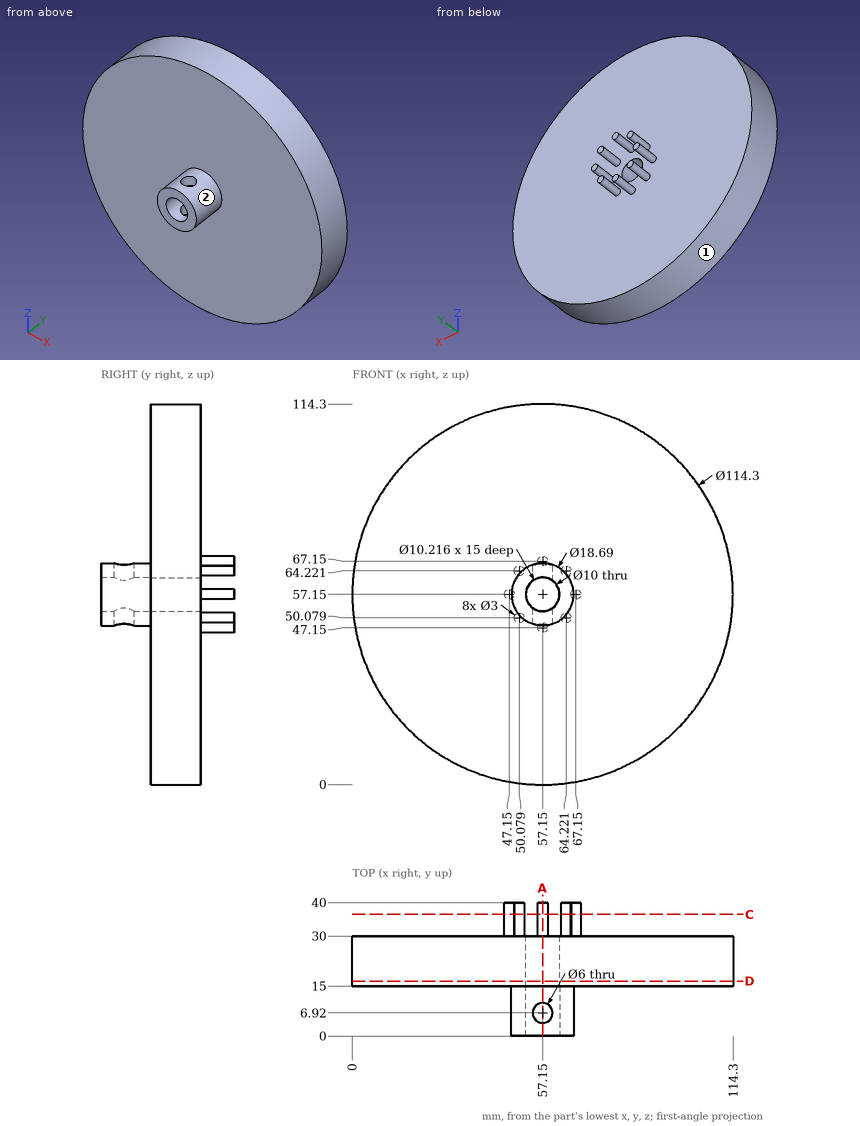
Print and shaded views of the part. All mm, measured from the part's lowest x, y and z. A direction names the side the tool comes from. Round coordinates to 2 decimals unless told otherwise and drop trailing zeros. Write each loop counter-clockwise with the first axis right and the second up, starting at its lowest first coordinate (ties: lowest second). Pieces come first, ordered by that corner, then holes.
(1) Probe line 1 along Y through (x, z) = (57.15, 49.7); line 2 along Z through (x, y) = (57, 20); line 3 along X through (y, z) = (4, 57) (1 decimal). List the from-to ranges inside material, lowest first.
(2) 3-axis set-ups, long thin cutter, end or side, ignore diameter. For the marked faces 1 and 2: which of +Z, -Z, +X, -X, +Y, -Y reach the whole face in a straight line?
(3) Drop flat-ended pins along their axis: P1, Ø6, axis at x = 57.15, z = 57.15, coming from the +Y side; P2, Ø8, axis at x = 57.15, y = 6.92, coming from the -Z side (1 decimal); P3, Ø12, axis at y = 15.5, z = 95.5, coming from the +X side; P4, Ø2, axis at x = 61.5, z = 24, coming from the +Y side. Give the stop position or say it passes through.
(4) Slice it at C-C, the plane y = 36.5. Write the cut outline in (x, z).
(5) Slice it at A-A, the plane x = 57.15. Count the separate pieces of the cut face and the enclosed holes in it, and give its area (3 significant figures).
(6) Slice it at D-D, the plane y = 16.5. Write the cut outline in (x, z).
From the geometry:
1. line 1: y = 0 to 3.92, 9.92 to 30
1. line 2: z = 0 to 52.15, 62.15 to 114.3
1. line 3: x = 47.8 to 52, 62.3 to 66.5
2. face 1: +Y, -Y
2. face 2: -Y
3. P1: passes through
3. P2: stops at z = 47.8
3. P3: stops at x = 104.26
3. P4: stops at y = 30
4. outline: circle Ø3 at (47.15, 57.15); circle Ø3 at (50.08, 50.08); circle Ø3 at (50.08, 64.22); circle Ø3 at (57.15, 47.15); circle Ø3 at (57.15, 67.15); circle Ø3 at (64.22, 50.08); circle Ø3 at (64.22, 64.22); circle Ø3 at (67.15, 57.15)
5. separate pieces: 4
5. enclosed holes: 0
5. area: 1,700 mm2
6. outline: circle Ø114.3 at (57.15, 57.15); hole circle Ø10 at (57.15, 57.15)
